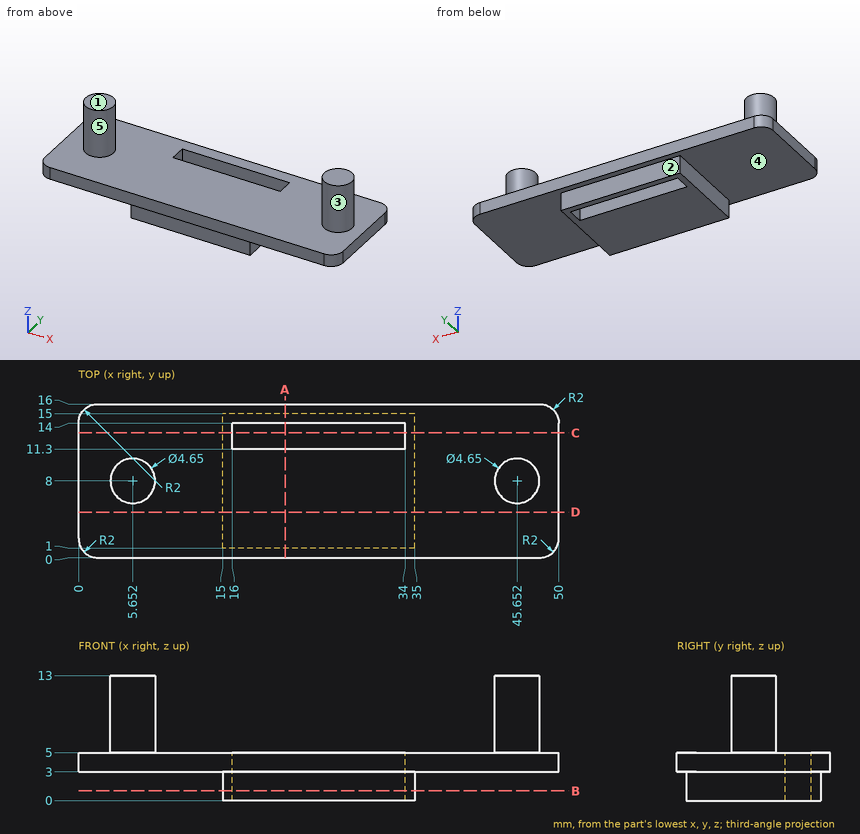
Can you work these out from the drawing? Everything is in mm from the part's minimum corner. A direction names the side the tool comes from. Give positions to 0.01 mm unless a question says otherwise; leave off trailing zeros. Write each loop counter-clockwise with the first axis right and the second up, starting at its lowest first coordinate (ties: lowest second). Pieces come first, ordered by that corner, then holes. Notation, with made-up numbers: (-18, 42.25) -> (35, 42.25) arc R32 cw to (35, 75.25) -> close; hole circle Ø6 at (-38.5, -5). An arc over 180 degrees is marked (long way). Write each question's results on one line, items separated by ' | '.
Item 1: On a 3-axis mill with a long thin cutter (end or side, diameter ignored), from which of +Z, -Z, +X, -X, +Y, -Y can I reach the whole of each face in a straight line? I mean the marked faces 1, 2 and 3. Say none if no direction works.
Output:
face 1: +Z, +X, -X, +Y, -Y | face 2: -Z, +X, -X, +Y | face 3: +Z
Item 2: Suppose I cut it at D-D on y = 4.75. Write out the boundary of the cut face in (x, z), plus the area to 3 significant figures.
Output:
outline: (0, 3) -> (15, 3) -> (15, 0) -> (35, 0) -> (35, 3) -> (50, 3) -> (50, 5) -> (0, 5) -> close | area: 160 mm^2
Item 3: We'd pull the mould along X, two halves only. Please class the marked faces 4 and 5: pulls with the +X half, pulls with the -X half, needs draft (parallel to the pull), parting line crosses it, or undercut.
Output:
face 4: needs draft | face 5: undercut
Item 4: Suppose I cut it at A-A on x = 21.5. Write out the boundary of the cut face in (y, z), plus the area to 3 significant figures.
Output:
outline: (0, 3) -> (1, 3) -> (1, 0) -> (11.3, 0) -> (11.3, 5) -> (0, 5) -> close; (14, 0) -> (15, 0) -> (15, 3) -> (16, 3) -> (16, 5) -> (14, 5) -> close | area: 60.5 mm^2
Item 5: If I drill on L1, parallel to Y at x = 32.5, z = 4.25; L2, parallel to X at y = 8, z = 1; L3, parallel to Z at x = 12.5, y = 14.5, over which ranges is the centre line in solid material (lowest first)?
Output:
L1: y = 0 to 11.3, 14 to 16 | L2: x = 15 to 35 | L3: z = 3 to 5
Item 6: Suppose I cut it at B-B on z = 1. Write out the boundary of the cut face in (x, y), plus the area to 3 significant figures.
Output:
outline: (15, 1) -> (35, 1) -> (35, 15) -> (15, 15) -> close; hole (16, 11.3) -> (34, 11.3) -> (34, 14) -> (16, 14) -> close | area: 231 mm^2
Item 7: For pin 1 Ø1.5 at (x, y) = (10, 6.5) entering from +Z; pin 2 Ø5 at (x, z) = (23, 8.5) entering from +Y; pin 3 Ø3 at (y, z) = (5, 11) entering from -X (1 decimal); pin 4 Ø1.5 at (y, z) = (9, 2) entering from -X, each with a flat end and sliding along its axis, tell me the tip position at first contact or that it passes through.
Output:
pin 1: stops at z = 5 | pin 2: passes through | pin 3: stops at x = 3.9 | pin 4: stops at x = 15
Item 8: Suppose I cut it at C-C on y = 13. Write out the boundary of the cut face in (x, z), plus the area to 3 significant figures.
Output:
outline: (0, 3) -> (15, 3) -> (15, 0) -> (16, 0) -> (16, 5) -> (0, 5) -> close; (34, 0) -> (35, 0) -> (35, 3) -> (50, 3) -> (50, 5) -> (34, 5) -> close | area: 70.0 mm^2
